Model file for the job. Use its own axes, mm. A direction names the side the tool comes from. Give positions to 0.01 mm unless a question says otherwise; leave off trailing zeros. Write each loop counter-clockwise with the first axis right and the second up, starting at its lowest first coordinate (ties: lowest second). Pieces come first, ordered by that corner, then holes. Notation, with made-up numbers: (65, 26.5) - (89, 26.5) arc R17 cw to (89, 55.5) - close; hole circle Ø11 at (52.5, -25.75). An arc over 180 degrees is marked (long way). One line per item, written item: value. Start each with the question number.
(1) Cut at D-D, the plane y = 3.55. State how many separate pieces and enclosed holes the cut face has, and give its area (3 significant figures).
(2) Cut at C-C, the plane x = 9. List the corners of the cut face in (y, z), and give its area (3 significant figures).
(3) Probe L1, parallel to Z at x = -29.5, y = 4.55; L2, parallel to Z at x = 50, y = 3.75; L3, parallel to X at y = 4.65, z = 14 (3 decimals). List the from-to ranges inside material, lowest first.
(4) Cut at B-B, the plane z = -20. List the corners of the cut face in (x, y).
(5) 3-axis set-ups, long thin cutter, end or side, ignore diameter. For faces 4 (the face through (1, 3, 48)), 5 (the face through (-29.075, 3, 30)): which of +Z, -Z, +X, -X, +Y, -Y reach the whole face in a straight line?
(6) Cut at A-A, the plane x = -50. List the corners of the cut face in (y, z), and give its area (3 significant figures).
(7) Mould opens along X. For faces 1 (the face through (14, 6, 1)), 2 (the face through (15.15, 3, 9)), 3 (the face through (-57, 3, 47)) say: pulls with the +X half, pulls with the -X half, needs draft (parallel to the pull), parting line crosses it, or undercut.
Autodesk Inventor part; units mm, degrees
ref_plane "YZ Plane" through (0, 0, 0) normal (1, 0, 0) x (0, 1, 0)
ref_plane "XZ Plane" through (0, 0, 0) normal (0, 1, 0) x (-1, 0, 0)
ref_plane "XY Plane" through (0, 0, 0) normal (0, 0, 1) x (1, 0, 0)
sketch "Sketch1" plane through (0, 0, 0) normal (0, 1, 0) x (-1, 0, 0)
  line L0 (54, -48) -> (-54, -48)
  line L1 (-59, -43) -> (-59, 43)
  line L2 (-54, 48) -> (54, 48)
  line L3 (59, 43) -> (59, -43)
  line L4 (50, -35) -> (-50, -35) construction
  line L5 (-50, -35) -> (-50, 35) construction
  line L6 (-50, 35) -> (50, 35) construction
  line L7 (50, 35) -> (50, -35) construction
  arc A0 (59, 43) -> (54, 48) centre (54, 43) ccw
  arc A1 (-54, 48) -> (-59, 43) centre (-54, 43) ccw
  arc A2 (-59, -43) -> (-54, -48) centre (-54, -43) ccw
  arc A3 (54, -48) -> (59, -43) centre (54, -43) ccw
  circle A4 centre (50, -35) radius 3.4
  circle A5 centre (50, 35) radius 3.4
  circle A6 centre (-50, -35) radius 3.4
  circle A7 centre (-50, 35) radius 3.4
  line L8 (0, -20) -> (0, 20) construction
  line L9 (25, -20) -> (25, 20) construction
  line L10 (-25, 20) -> (-25, -20) construction
  arc A8 (-25, -20) -> (25, -20) centre (0, -20) ccw construction
  arc A9 (25, 20) -> (-25, 20) centre (0, 20) ccw construction
  circle A10 centre (0, -20) radius 22.5
  circle A11 centre (50, -35) radius 9.5 construction
  circle A12 centre (-50, -35) radius 9.5 construction
  circle A13 centre (50, 35) radius 9.5 construction
  circle A14 centre (-50, 35) radius 9.5 construction
  line L11 (35, -35) -> (29, -35) construction
  line L12 (29, -35) -> (29, 35) construction
  line L13 (29, 35) -> (35, 35) construction
  line L14 (35, 35) -> (35, -35) construction
  line L15 (35, 6.4) -> (-35, 6.4) construction
  line L16 (-35, 12.4) -> (35, 12.4) construction
  line L17 (35, 12.4) -> (35, 6.4) construction
  line L18 (-25, -20) -> (-25, 20) construction
  line L19 (4.85, 6.475) -> (-4.85, 6.475)
  line L20 (-4.85, 6.475) -> (-4.85, 12.325)
  line L21 (-4.85, 12.325) -> (4.85, 12.325)
  line L22 (4.85, 12.325) -> (4.85, 6.475)
  line L23 (0, 6.4) -> (0, 12.4) construction
  line L24 (34.925, -34.85) -> (29.075, -34.85)
  line L25 (29.075, -34.85) -> (29.075, -25.15)
  line L26 (29.075, -25.15) -> (34.925, -25.15)
  line L27 (34.925, -25.15) -> (34.925, -34.85)
  line L28 (34.925, -14.85) -> (29.075, -14.85)
  line L29 (34.925, -5.15) -> (34.925, -14.85)
  line L30 (29.075, -5.15) -> (34.925, -5.15)
  line L31 (29.075, -14.85) -> (29.075, -5.15)
  line L32 (34.925, 5.15) -> (29.075, 5.15)
  line L33 (34.925, 14.85) -> (34.925, 5.15)
  line L34 (29.075, 14.85) -> (34.925, 14.85)
  line L35 (29.075, 5.15) -> (29.075, 14.85)
  line L36 (34.925, 25.15) -> (29.075, 25.15)
  line L37 (34.925, 34.85) -> (34.925, 25.15)
  line L38 (29.075, 34.85) -> (34.925, 34.85)
  line L39 (29.075, 25.15) -> (29.075, 34.85)
  line L40 (-35, -35) -> (-29, -35) construction
  line L41 (-29, -35) -> (-29, 35) construction
  line L42 (-29, 35) -> (-35, 35) construction
  line L43 (-35, 35) -> (-35, -35) construction
  line L44 (-35, 12.4) -> (-35, 6.4) construction
  line L45 (-34.925, -34.85) -> (-29.075, -34.85)
  line L46 (-29.075, -34.85) -> (-29.075, -25.15)
  line L47 (-29.075, -25.15) -> (-34.925, -25.15)
  line L48 (-34.925, -25.15) -> (-34.925, -34.85)
  line L49 (-34.925, -14.85) -> (-29.075, -14.85)
  line L50 (-34.925, -5.15) -> (-34.925, -14.85)
  line L51 (-29.075, -5.15) -> (-34.925, -5.15)
  line L52 (-29.075, -14.85) -> (-29.075, -5.15)
  line L53 (-34.925, 5.15) -> (-29.075, 5.15)
  line L54 (-34.925, 14.85) -> (-34.925, 5.15)
  line L55 (-29.075, 14.85) -> (-34.925, 14.85)
  line L56 (-29.075, 5.15) -> (-29.075, 14.85)
  line L57 (-34.925, 25.15) -> (-29.075, 25.15)
  line L58 (-34.925, 34.85) -> (-34.925, 25.15)
  line L59 (-29.075, 34.85) -> (-34.925, 34.85)
  line L60 (-29.075, 25.15) -> (-29.075, 34.85)
  line L61 (24.85, 6.475) -> (15.15, 6.475)
  line L62 (24.85, 12.325) -> (24.85, 6.475)
  line L63 (20, 6.4) -> (20, 12.4) construction
  line L64 (15.15, 12.325) -> (24.85, 12.325)
  line L65 (15.15, 6.475) -> (15.15, 12.325)
  line L66 (-15.15, 6.475) -> (-24.85, 6.475)
  line L67 (-15.15, 12.325) -> (-15.15, 6.475)
  line L68 (-20, 6.4) -> (-20, 12.4) construction
  line L69 (-24.85, 12.325) -> (-15.15, 12.325)
  line L70 (-24.85, 6.475) -> (-24.85, 12.325)
  line L71 (4.85, 6.475) -> (-4.85, 6.475)
  line L72 (4.85, 12.325) -> (4.85, 6.475)
  line L73 (0, 6.4) -> (0, 12.4) construction
  line L74 (-4.85, 12.325) -> (4.85, 12.325)
  line L75 (-4.85, 6.475) -> (-4.85, 12.325)
  point P0 (0, 0)
  point P1 (-59, 0)
  point P2 (0, -48)
  point P3 (0, -35)
  point P4 (-50, 0)
  point P5 (0, 0)
  point P6 (32, -35)
  point P7 (-4.85, 9.4)
  point P8 (4.85, 9.4)
  point P9 (0, 6.475)
  point P10 (32, -25.15)
  point P11 (32, -30)
  point P12 (29.075, -30)
  point P13 (32, -34.85)
  point P14 (32, -35)
  point P15 (29, 0)
  point P16 (32, -14.85)
  point P17 (32, -5.15)
  point P18 (29.075, -10)
  point P19 (32, -10)
  point P20 (32, 5.15)
  point P21 (32, 14.85)
  point P22 (29.075, 10)
  point P23 (32, 10)
  point P24 (32, 25.15)
  point P25 (32, 34.85)
  point P26 (29.075, 30)
  point P27 (32, 30)
  point P28 (-32, -35)
  point P29 (-32, -25.15)
  point P30 (-32, -30)
  point P31 (-29.075, -30)
  point P32 (-32, -34.85)
  point P33 (-32, -35)
  point P34 (-29, 0)
  point P35 (-32, -14.85)
  point P36 (-32, -5.15)
  point P37 (-29.075, -10)
  point P38 (-32, -10)
  point P39 (-32, 5.15)
  point P40 (-32, 14.85)
  point P41 (-29.075, 10)
  point P42 (-32, 10)
  point P43 (-32, 25.15)
  point P44 (-32, 34.85)
  point P45 (-29.075, 30)
  point P46 (-32, 30)
  point P47 (35, 9.4)
  point P48 (35, 0)
  point P49 (20, 6.475)
  point P50 (24.85, 9.4)
  point P51 (15.15, 9.4)
  point P52 (-20, 6.475)
  point P53 (-15.15, 9.4)
  point P54 (-24.85, 9.4)
  point P55 (0, 6.475)
  point P56 (4.85, 9.4)
  point P57 (-4.85, 9.4)
  dimension "d0" = 96
  dimension "d1" = 118
  dimension "d2" = 70
  dimension "d3" = 100
  dimension "d4" = 5
  dimension "d5" = 6.8
  dimension "d6" = 6.8
  dimension "d8" = 6.8
  dimension "d10" = 6.8
  dimension "d13" = 25
  dimension "d14" = 40
  dimension "d17" = 45
  dimension "d19" = 19
  dimension "d22" = 100
  dimension "d25" = 70
  dimension "d28" = 6
  dimension "d29" = 6
  dimension "d30" = 26.4
  dimension "d31" = 15
  dimension "d41" = 5.85
  dimension "d42" = 9.7
  dimension "d54" = 5.85
  dimension "d55" = 9.7
  dimension "d56" = 30
  dimension "d59" = 20
  dimension "d64" = 9.4
  dimension "d67" = 20
  dimension "d70" = 20
extrude "Extrusion1" add sketch "Sketch1" along normal blind 6
equation "\"d0\" = moduleHeight"
equation "\"d1\" = moduleWidth"
equation "\"d2\" = moduleMountH"
equation "\"d3\" = moduleMountW"
equation "\"d4\" = moduleCornerR"
equation "\"d5\" = moduleMountD"
equation "\"d6\" = moduleMountD"
equation "\"d8\" = moduleMountD"
equation "\"d10\" = moduleMountD"
equation "\"d13\" = moduleOpeningR"
equation "\"d14\" = moduleOpeningH"
equation "\"d17\" = openingMFC"
equation "\"d19\" = moduleMountClearance"
equation "\"d28\" = thickness"
equation "\"d29\" = thickness"
equation "\"d30\" = 0.5 * actuatorH + thickness"
equation "\"d31\" = supportSpacingFromMounting"
equation "\"d41\" = fingerholeH"
equation "\"d54\" = fingerholeH"
equation "\"d15\" = thickness"
equation "\"moduleWidth\" = 118"
equation "\"moduleHeight\" = 96"
equation "\"moduleMountW\" = 100"
equation "\"moduleMountH\" = 70"
equation "\"moduleMountD\" = 6.8"
equation "\"moduleCornerR\" = 5"
equation "\"moduleOpeningR\" = 25"
equation "\"moduleOpeningH\" = 40"
equation "\"thickness\" = 6"
equation "\"kerf\" = 0.15"
equation "\"fingerholeW\" = fingerW - 2 * kerf"
equation "\"fingerholeH\" = thickness - kerf"
equation "\"moduleMountClearance\" = 19"
equation "\"actuatorW\" = 28"
equation "\"actuatorH\" = 40.8"
equation "\"openingMFC\" = 45"
equation "\"supportXW\" = -2 * thickness + moduleMountW - 2 * supportSpacingFromMounting + kerf"
equation "\"supportSpacingFromMounting\" = 15"
equation "\"supportsCTCZ\" = 9.4"
properties part number "Module_base_MFC"
Answers follow:
1. separate pieces: 1
1. enclosed holes: 16
1. area: 8,950 mm²
2. outline: (0, -48) - (6, -48) - (6, -40.62) - (0, -40.62) - close; (0, 0.62) - (6, 0.62) - (6, 48) - (0, 48) - close
2. area: 329 mm²
3. L1: z = -48 to -34.85, -25.15 to -14.85, -5.15 to 5.15, 14.85 to 25.15, 34.85 to 48
3. L2: z = -48 to -38.4, -31.6 to 31.6, 38.4 to 48
3. L3: x = -59 to -34.925, -29.075 to 29.075, 34.925 to 59
4. outline: (-59, 0) - (-22.5, 0) - (-22.5, 6) - (-59, 6) - close; (22.5, 0) - (59, 0) - (59, 6) - (22.5, 6) - close
5. face 4: +Z, +X, -X, +Y, -Y
5. face 5: +Y, -Y
6. outline: (0, -48) - (6, -48) - (6, -38.4) - (0, -38.4) - close; (0, -31.6) - (6, -31.6) - (6, 31.6) - (0, 31.6) - close; (0, 38.4) - (6, 38.4) - (6, 48) - (0, 48) - close
6. area: 494 mm²
7. face 1: needs draft
7. face 2: undercut
7. face 3: pulls with the -X half
